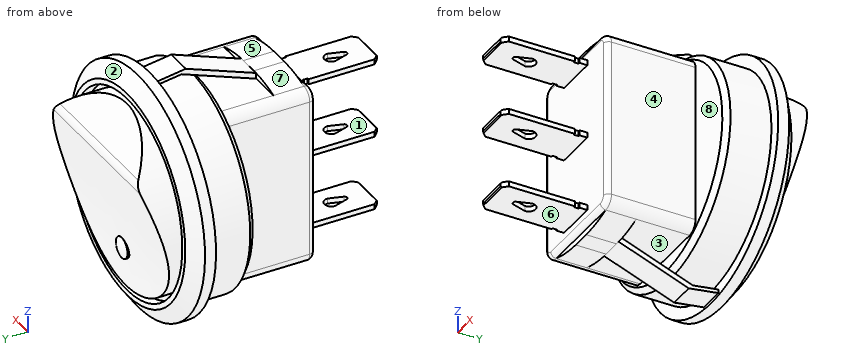
```python
from build123d import *

# Parameters (mm, degrees)
CUT_EXTRUDE1_DEPTH       = 10
CUT_EXTRUDE1_DEPTH_BACK  = 10
SKETCH4_R                = 9.5
SKETCH4_R_2              = 9
CUT_EXTRUDE2_DEPTH       = 1
BOSS_EXTRUDE1_DEPTH      = 5.25
BOSS_EXTRUDE1_DEPTH_BACK = 5.25
SKETCH5_W                = 17.1
SKETCH5_H                = 8.5
FILLET1_R                = 1
FILLET2_R                = 0.5
BOSS_EXTRUDE2_DEPTH      = 2
BOSS_EXTRUDE2_DEPTH_BACK = 2
CUT_EXTRUDE4_REACH       = 33.935
SKETCH7_W                = 0.15198881
SKETCH7_H                = 0.437250331
SKETCH8_R                = 1
BOSS_EXTRUDE4_DEPTH      = 0.5
DOME1_FACE_RADIUS        = 1
DOME1_HEIGHT             = 0.25
BOSS_EXTRUDE5_DEPTH      = 1.25
SKETCH11_W               = 8.5
SKETCH11_H               = 2.901212209
BOSS_EXTRUDE6_DEPTH      = 0.55
FILLET3_R                = 10.5
MIRROR2_START            = -14.5
MIRROR2_DEPTH            = 2.901212209


# Read off the part's stored shape, not the designer's step: Mirror2
with BuildPart() as part:
    # Sketch1 → Revolve1 (revolve)
    with BuildSketch(Plane(origin=(0, 0, 0), x_dir=(0, 0, -1), z_dir=(1, 0, 0))):
        Polygon((0, -6.5), (-9.85, -6.5), (-10.35, -6), (-10.35, -2.1), (-11.5, -2.1), (-11.5, -1.05), (-10, 0), (-9, 0), (-9, 3), (0, 3), (0, 0), align=None)
    revolve(axis=Axis((0, 0, 0), (0, -1, 0)))

    # Sketch3 → Cut-Extrude1 (cut, two sides: drawn at the far end of the back side and taken through both)
    with BuildSketch(Plane(origin=(0, 0, 0), x_dir=(0, 0, -1), z_dir=(1, 0, 0)).offset(-CUT_EXTRUDE1_DEPTH_BACK)):
        with BuildLine():
            Line((-9, 0), (-6.004871006, 2.642395133))
            ThreePointArc((-6.004871006, 2.642395133), (-5.571055004, 2.86623052), (-5.082965507, 2.858030108))
            add(Edge.make_bspline(
                [(9, 0.1), (3.500957761, 0.065162529), (-0.63708622, 1.659275419), (-5.082965507, 2.858030108)],
                knots=[0, 0, 0, 0, 0.851151632, 0.851151632, 0.851151632, 0.851151632], degree=3))
            Line((9, 0.1), (9, 3))
            Line((9, 3), (-9, 3))
            Line((-9, 3), (-9, 0))
        make_face()
    extrude(amount=CUT_EXTRUDE1_DEPTH + CUT_EXTRUDE1_DEPTH_BACK, mode=Mode.SUBTRACT)

    # Sketch4 → Cut-Extrude2 (cut)
    with BuildSketch(Plane(origin=(0, 0, 0), x_dir=(1, 0, 0), z_dir=(0, 1, 0))):
        with Locations(Location((0, 0, 0), (0, 0, 270))):
            Circle(SKETCH4_R)
        with Locations(Location((0, 0, 0), (0, 0, 270))):
            Circle(SKETCH4_R_2, mode=Mode.SUBTRACT)
    extrude(amount=-CUT_EXTRUDE2_DEPTH, mode=Mode.SUBTRACT)

    # Sketch5 → Boss-Extrude1 (add, two sides: drawn at the far end of the back side and taken through both)
    with BuildSketch(Plane(origin=(0, 0, 0), x_dir=(0, 0, -1), z_dir=(1, 0, 0)).offset(-BOSS_EXTRUDE1_DEPTH_BACK)):
        with Locations((0, -10.75)):
            Rectangle(SKETCH5_W, SKETCH5_H)
    extrude(amount=BOSS_EXTRUDE1_DEPTH + BOSS_EXTRUDE1_DEPTH_BACK)

    # Fillet1
    # the kernel refuses this fillet: 1 mm, written as the material it takes off along each edge
    with BuildSketch(Plane(origin=(-5.25, -17.5, 8.55), x_dir=(1, 0, 0), z_dir=(0, 1, 0)), Plane(origin=(5.25, -6.5, -8.55), x_dir=(0, 0, 1), z_dir=(0, -1, 0))) as fillet1_piece_1:
        with BuildLine():
            CenterArc((FILLET1_R, FILLET1_R), FILLET1_R, 180, 90)
            Line((0, FILLET1_R), (0, 0))
            Line((0, 0), (FILLET1_R, 0))
        make_face()
    extrude(amount=11, mode=Mode.SUBTRACT)
    with BuildSketch(Plane(origin=(-5.25, -6.5, -8.55), x_dir=(0, 0, 1), z_dir=(0, -1, 0)), Plane(origin=(5.25, -17.5, 8.55), x_dir=(-1, 0, 0), z_dir=(0, 1, 0))) as fillet1_piece_2:
        with BuildLine():
            CenterArc((FILLET1_R, -FILLET1_R), FILLET1_R, 90, 90)
            Line((0, -FILLET1_R), (0, 0))
            Line((0, 0), (FILLET1_R, 0))
        make_face()
    extrude(amount=11, mode=Mode.SUBTRACT)

    # Fillet2
    fillet2_edges = [part.edges().sort_by_distance(p)[0] for p in [
        (0, -15, 8.55),
        (0, -15, -8.55),
        (5.25, -15, 0),
        (-5.25, -15, 0),
        (4.957106781, -15, 8.257106781),
        (4.957106781, -15, -8.257106781),
        (-4.957106781, -15, -8.257106781),
        (-4.957106781, -15, 8.257106781),
    ]]
    fillet(fillet2_edges, radius=FILLET2_R)

    # Sketch6 → Boss-Extrude2 (add, two sides: drawn at the far end of the back side and taken through both)
    with BuildSketch(Plane(origin=(0, 0, 0), x_dir=(0, 0, -1), z_dir=(1, 0, 0)).offset(-BOSS_EXTRUDE2_DEPTH_BACK)):
        Polygon((0.25, -15), (-0.25, -15), (-0.25, -22.9), (-0.15, -23), (0.15, -23), (0.25, -22.9), align=None)
        Polygon((-7.337194576, -23), (-7.037194576, -23), (-6.937194576, -22.9), (-6.937194576, -15), (-7.437194576, -15), (-7.437194576, -22.9), align=None)
        Polygon((7.437194576, -22.9), (7.337194576, -23), (7.037194576, -23), (6.937194576, -22.9), (6.937194576, -15), (7.437194576, -15), align=None)
    extrude(amount=BOSS_EXTRUDE2_DEPTH + BOSS_EXTRUDE2_DEPTH_BACK)

    # Cut-Extrude4: up to this face of the body (flat: up to its plane)
    cut_extrude4_end = Plane(part.part.faces().sort_by_distance((0, -18.95, 7.437194576))[0])
    # Sketch7 → Cut-Extrude4 (cut, up to the picked face)
    with BuildSketch(Plane(origin=(0, 0, -7.437194576), x_dir=(-1, 0, 0), z_dir=(0, 0, -1)), mode=Mode.PRIVATE) as cut_extrude4_sk1:
        Polygon((1.48452642, -23), (2, -22.48452642), (2, -23), align=None)
    cut_extrude4_tool1 = split(extrude(cut_extrude4_sk1.sketch, amount=-CUT_EXTRUDE4_REACH, mode=Mode.PRIVATE), bisect_by=cut_extrude4_end, keep=Keep.BOTH, mode=Mode.PRIVATE)
    # Sketch7 → Cut-Extrude4 (cut, up to the picked face)
    with BuildSketch(Plane(origin=(0, 0, -7.437194576), x_dir=(-1, 0, 0), z_dir=(0, 0, -1)), mode=Mode.PRIVATE) as cut_extrude4_sk2:
        with Locations((1.924005595, -15.976692476)):
            Rectangle(SKETCH7_W, SKETCH7_H)
    cut_extrude4_tool2 = split(extrude(cut_extrude4_sk2.sketch, amount=-CUT_EXTRUDE4_REACH, mode=Mode.PRIVATE), bisect_by=cut_extrude4_end, keep=Keep.BOTH, mode=Mode.PRIVATE)
    # Sketch7 → Cut-Extrude4 (cut, up to the picked face)
    with BuildSketch(Plane(origin=(0, 0, -7.437194576), x_dir=(-1, 0, 0), z_dir=(0, 0, -1)), mode=Mode.PRIVATE) as cut_extrude4_sk3:
        with Locations((-1.924005595, -15.976692476)):
            Rectangle(SKETCH7_W, SKETCH7_H)
    cut_extrude4_tool3 = split(extrude(cut_extrude4_sk3.sketch, amount=-CUT_EXTRUDE4_REACH, mode=Mode.PRIVATE), bisect_by=cut_extrude4_end, keep=Keep.BOTH, mode=Mode.PRIVATE)
    # Sketch7 → Cut-Extrude4 (cut, up to the picked face)
    with BuildSketch(Plane(origin=(0, 0, -7.437194576), x_dir=(-1, 0, 0), z_dir=(0, 0, -1)), mode=Mode.PRIVATE) as cut_extrude4_sk4:
        Polygon((-1.48452642, -23), (-2, -22.48452642), (-2, -23), align=None)
    cut_extrude4_tool4 = split(extrude(cut_extrude4_sk4.sketch, amount=-CUT_EXTRUDE4_REACH, mode=Mode.PRIVATE), bisect_by=cut_extrude4_end, keep=Keep.BOTH, mode=Mode.PRIVATE)
    # Sketch7 → Cut-Extrude4 (cut, up to the picked face)
    with BuildSketch(Plane(origin=(0, 0, -7.437194576), x_dir=(-1, 0, 0), z_dir=(0, 0, -1)), mode=Mode.PRIVATE) as cut_extrude4_sk5:
        with BuildLine():
            Line((-0.652188184, -19.474698282), (-0.238643365, -20.799500715))
            ThreePointArc((-0.238643365, -20.799500715), (0, -20.975006794), (0.238643365, -20.799500715))
            Line((0.238643365, -20.799500715), (0.652188184, -19.474698282))
            ThreePointArc((0.652188184, -19.474698282), (0, -18.822510099), (-0.652188184, -19.474698282))
        make_face()
    cut_extrude4_tool5 = split(extrude(cut_extrude4_sk5.sketch, amount=-CUT_EXTRUDE4_REACH, mode=Mode.PRIVATE), bisect_by=cut_extrude4_end, keep=Keep.BOTH, mode=Mode.PRIVATE)
    add(cut_extrude4_tool1.solids().sort_by(Axis((-1.828175, -22.828175, -7.437195), (0, 0, 1)))[0], mode=Mode.SUBTRACT)
    add(cut_extrude4_tool2.solids().sort_by(Axis((-1.924006, -15.976692, -7.437195), (0, 0, 1)))[0], mode=Mode.SUBTRACT)
    add(cut_extrude4_tool3.solids().sort_by(Axis((1.924006, -15.976692, -7.437195), (0, 0, 1)))[0], mode=Mode.SUBTRACT)
    add(cut_extrude4_tool4.solids().sort_by(Axis((1.828175, -22.828175, -7.437195), (0, 0, 1)))[0], mode=Mode.SUBTRACT)
    add(cut_extrude4_tool5.solids().sort_by(Axis((0, -19.768855, -7.437195), (0, 0, 1)))[0], mode=Mode.SUBTRACT)

    # Sketch8 → Boss-Extrude4 (add)
    with BuildSketch(Plane(origin=(0, 0, 0), x_dir=(1, 0, 0), z_dir=(0, 1, 0))):
        with Locations(Location((0, 5.153544254, 0), (0, 0, 90))):
            Circle(SKETCH8_R)
    extrude(amount=BOSS_EXTRUDE4_DEPTH)

    # Dome1: a dome of height H over a round flat face of radius A is a cap of a sphere of radius (A * A + H * H) / (2 * H)
    dome1_r = (DOME1_FACE_RADIUS * DOME1_FACE_RADIUS + DOME1_HEIGHT * DOME1_HEIGHT) / (2 * DOME1_HEIGHT)
    dome1_base = Plane((0, 0.5, -5.153544254), z_dir=(0, 1, 0))
    with Locations(dome1_base.offset(DOME1_HEIGHT - dome1_r)):
        dome1_ball = Sphere(dome1_r, mode=Mode.PRIVATE)
    add(split(dome1_ball, bisect_by=dome1_base, keep=Keep.TOP, mode=Mode.PRIVATE))

    # Sketch9 → Boss-Extrude5 (add, symmetric)
    with BuildSketch(Plane(origin=(0, 0, 0), x_dir=(0, 0, -1), z_dir=(1, 0, 0))):
        Polygon((11.189766079, -2.1), (11.603464839, -4.916902693), (8.55, -13.011373866), (8.55, -11.511373866), (11.189766079, -4.513582322), (10.835300156, -2.1), align=None)
    boss_extrude5 = extrude(amount=BOSS_EXTRUDE5_DEPTH, both=True)

    # Mirror1: Boss-Extrude5 across plane
    add(boss_extrude5.mirror(Plane.XY))

    # Sketch11 → Boss-Extrude6 (add)
    with BuildSketch(Plane(origin=(0, 0, -8.55), x_dir=(-1, 0, 0), z_dir=(0, 0, -1))):
        with Locations((0, -13.049393896)):
            Rectangle(SKETCH11_W, SKETCH11_H)
    extrude(amount=BOSS_EXTRUDE6_DEPTH)

    # Fillet3
    # the kernel refuses this fillet: 10.5 mm, written as the material it takes off along each edge
    with BuildSketch(Plane(origin=(4.25, -22.884323169, -9.1), x_dir=(-1.1142601992564705e-12, 0, 1.0), z_dir=(0, 1, 0)), Plane(origin=(-4.25, -11.598787791, -9.1), x_dir=(1.1142601992564705e-12, 0, 1.0), z_dir=(0, -1, 0))) as fillet3_piece_1:
        with BuildLine():
            CenterArc((10.5, -3.353729268), FILLET3_R, 161.37318815, 18.62681185)
            Line((0, -3.353729268), (0, 0))
            Line((0, 0), (0.55, 0))
        make_face()
    extrude(amount=11.285535378, mode=Mode.SUBTRACT)

    # Mirror2 outline → Mirror2 (add)
    with BuildSketch(Plane(origin=(0, 0, 0), x_dir=(1, 0, 0), z_dir=(0, 1, 0)).offset(MIRROR2_START)):
        with BuildLine():
            Line((-0.896270732, -9.1), (0.896270732, -9.1))
            ThreePointArc((0.896270732, -9.1), (2.595535279, -8.961587716), (4.25, -8.55))
            Line((4.25, -8.55), (-4.25, -8.55))
            ThreePointArc((-4.25, -8.55), (-2.595535279, -8.961587716), (-0.896270732, -9.1))
        make_face()
    extrude(amount=MIRROR2_DEPTH)


solid = part.part
```
The model under review builds one solid part; all positions refer to its coordinate system, in mm. Face numbers are marked on the shaded views. A direction names the side the tool comes from. Coordinates: 2 decimals unless noted, no trailing zeros. Write each loop counter-clockwise with the first axis right and the second up, starting at its lowest first coordinate (ties: lowest second). Pieces come first, ordered by that corner, then holes. Notation, with made-up numbers: (81.25, -5.75) - (136.25, -5.75) arc R14 ccw to (136.25, 4.25) - close; hole circle Ø6 at (-3, 33). An arc over 180 degrees is marked (long way). Answer in a Markdown table with one row per item. Add a question column.
Q1. To check wall thickness, follow line 1 along Z through (x, y) = (1.5, -18.5); line 2 along X through (y, z) = (-0.75, 0); line 3 along X through (y, z) = (-0.5, 0). State the ranges of each line that lie inside material, in increasing order. Write a range as from..to.
Q2. Clearance check with flat-ended pins moving along their axes: pin 1 (10 mm diameter, centred on x = 4.5, z = 4.5, fed in from +Y); pin 2 (6 mm diameter, centred on y = -20, z = -5.5, fed in from +X); pin 3 (10 mm diameter, centred on y = -4.5, z = -8.5, fed in from +X); pin 4 (1.5 mm diameter, centred on x = -0.5, y = -9.5, fed in from +Z). State where each tip first meets the part, or that it passes through.
Q3. Draft analysis for pull direction Z (two halves, no side actions). For the marked faces 1, 2, 3 and 4, state which applies: +Z half, -Z half, draft (parallel to the pull), parting line (faces both ways), or undercut.
Q4. For the marked faces 5, 6, 7 and 8, list the 3-axis set-ups (+Z, -Z, +X, -X, +Y, -Y) from which the entire face can be reached by the end or side of a thin tool; tool diameter is ignored.
Q5. Consider section B-B on y = -7. Give the boundary of the cut face in (x, z), then the cut area to 3 significant figures.
Q6. Consider section A-A on y = -18.25. Give the boundary of the cut face in (x, z), then the cut area to 3 significant figures.
Answers below:
| question | item | result |
|---|---|---|
| 1 | line 1 | -7.44..-6.94, -0.25..0.25, 6.94..7.44 |
| 1 | line 2 | -11.07..-9.5, -9..9, 9.5..11.07 |
| 1 | line 3 | -10.71..-9.5, -9..9, 9.5..10.71 |
| 2 | pin 1 | y = 2.89 |
| 2 | pin 2 | x = 2 |
| 2 | pin 3 | x = 10.74 |
| 2 | pin 4 | z = 10.16 |
| 3 | face 1 | undercut |
| 3 | face 2 | parting line |
| 3 | face 3 | undercut |
| 3 | face 4 | draft |
| 4 | face 5 | +Z, +X, -Y |
| 4 | face 6 | -Z, +X, -X, -Y |
| 4 | face 7 | +Z, -X, -Y |
| 4 | face 8 | none |
| 5 | outline | (-5.25, -7.55) arc R1 ccw to (-4.25, -8.55) - (4.25, -8.55) arc R1 ccw to (5.25, -7.55) - (5.25, 7.55) arc R1 ccw to (4.25, 8.55) - (-4.25, 8.55) arc R1 ccw to (-5.25, 7.55) - close; (-1.25, -10.82) - (1.25, -10.82) - (1.25, -10.25) - (-1.25, -10.25) - close; (-1.25, 10.25) - (1.25, 10.25) - (1.25, 10.82) - (-1.25, 10.82) - close |
| 5 | area | 182 mm² |
| 6 | outline | (-2, -7.44) - (2, -7.44) - (2, -6.94) - (-2, -6.94) - close; (-2, -0.25) - (2, -0.25) - (2, 0.25) - (-2, 0.25) - close; (-2, 6.94) - (2, 6.94) - (2, 7.44) - (-2, 7.44) - close |
| 6 | area | 6.00 mm² |
